from build123d import *

# Parameters (mm, degrees)
CONG_1_R = 5


with BuildPart() as part:
    # Esquisse1 → Révolution1 (revolve)
    with BuildSketch(Plane.XY):
        Polygon((0, 0), (-140, 0), (-140, 50), (-100, 50), (-100, 15), (0, 15), align=None)
    r_volution1 = revolve(axis=Axis((0, 0, 0), (-1, 0, 0)))

    # Symétrie1: Révolution1 across plane
    add(r_volution1.mirror(Plane(origin=(0, 0, 0), x_dir=(0, 0, 1), z_dir=(1, 0, 0))))

    # Congé1
    cong_1_edges = [part.edges().sort_by_distance(p)[0] for p in [
        (100, -50, 0),
        (140, -50, 0),
        (-140, -50, 0),
        (-100, -50, 0),
    ]]
    fillet(cong_1_edges, radius=CONG_1_R)


solid = part.part
The model under review builds one solid part; all positions refer to its coordinate system, in mm. A direction names the side the tool comes from. Coordinates: 2 decimals unless noted, no trailing zeros. Loops run counter-clockwise (first coordinate to the right, second up) from the corner with the lowest first, then second, coordinate; pieces in that order, holes last. Notation, with made-up numbers: (61.5, 4.5) -> (108.5, 4.5) arc R22 ccw to (108.5, 31.5) -> close; hole circle Ø1 at (-19, 55). An arc over 180 degrees is marked (long way). Use a Markdown table: item, result. Add a question column.
1. Add section D-D on x = -117. Write out the cut boundary in (y, z).
2. Draft analysis for pull direction X (two halves, no side actions). For faces 3 (the face through (-140, 1, -1)), 4 (the face through (140, 1, -1)), 5 (the face through (-100, -11, -11)), state which applies: pulls with the +X half, pulls with the -X half, needs draft (parallel to the pull), parting line crosses it, or undercut.
3. Machinability: for faces 1 (the face through (-1.4, -14.985, -0.66)), 2 (the face through (119.79, 47.69, -15.02)), which of the approach directions +Z, -Z, +X, -X, +Y, -Y give a long, thin tool a straight path to every point of the face, cutting with its end or side? Answer none if there is none.
4. To check wall thickness, follow line 1 (X direction, y = 32, z = 0); line 2 (Y direction, x = -57, z = 1); line 3 (Z direction, x = -41, y = -0.5). State the ranges of each line that lie inside material, in increasing order.
5. Add section A-A on y = 0. Write out the cut boundary in (x, z), plus the area to 3 significant figures.
6. Clearance check with flat-ended pins moving along their axes: pin 1 Ø3 at (x, z) = (-19, -9.5) entering from -Y; pin 2 Ø8 at (x, z) = (51, 22.5) entering from -Y; pin 3 Ø8 at (x, z) = (-27.5, 12.5) entering from +Y. State where each tip first meets the part, or that it passes through.
7. Add section C-C on x = -54.5. Write out the cut boundary in (y, z).
Returned:
| question | item | result |
|---|---|---|
| 1 | outline | circle Ø100 at (0, 0) |
| 2 | face 3 | pulls with the -X half |
| 2 | face 4 | pulls with the +X half |
| 2 | face 5 | undercut |
| 3 | face 1 | none |
| 3 | face 2 | +X, -X |
| 4 | line 1 | x = -140 to -100, 100 to 140 |
| 4 | line 2 | y = -14.97 to 14.97 |
| 4 | line 3 | z = -14.99 to 14.99 |
| 5 | outline | (-140, -45) arc R5 ccw to (-135, -50) -> (-105, -50) arc R5 ccw to (-100, -45) -> (-100, -15) -> (100, -15) -> (100, -45) arc R5 ccw to (105, -50) -> (135, -50) arc R5 ccw to (140, -45) -> (140, 45) arc R5 ccw to (135, 50) -> (105, 50) arc R5 ccw to (100, 45) -> (100, 15) -> (-100, 15) -> (-100, 45) arc R5 ccw to (-105, 50) -> (-135, 50) arc R5 ccw to (-140, 45) -> close |
| 5 | area | 14,000 mm² |
| 6 | pin 1 | stops at y = -12.69 |
| 6 | pin 2 | passes through |
| 6 | pin 3 | stops at y = 12.36 |
| 7 | outline | circle Ø30 at (0, 0) |
